CAD build for the part. Positions are in the model's coordinates, mm. A direction names the side the tool comes from. Give positions to 0.01 mm unless a question says otherwise; leave off trailing zeros. Loops run counter-clockwise (first coordinate to the right, second up) from the corner with the lowest first, then second, coordinate; pieces in that order, holes last.
Item 1: Drop flat-ended pins along their axis: P1, Ø1, axis at y = 27, z = -35, coming from the -X side; P2, Ø12, axis at x = 11, y = 132.5, coming from the -Z side; P3, Ø8, axis at x = 11, y = 55, coming from the -Z side. Give the stop position or say it passes through.
Item 2: Probe probe 1 along X at (y, z) = (36, -101.5); probe 2 along Z at (x, y) = (22, 121); probe 3 along Z at (x, y) = (11, 14.5). List the from-to ranges inside material, lowest first.
Item 3: Saw through at A-A on x = 14.25. Give the cut face in (y, z).
Item 4: Saw through at C-C on z = -15. Give the cut face in (x, y).
Item 5: Saw through at D-D on y = 35. Give the cut face in (x, z), plus the area to 3 significant figures.
Item 6: Which spindle directions (+Z, -Z, +X, -X, +Y, -Y) get a long thin tool onto all of the face, cutting with end or side? Do faces 1 (the cylindrical face through (14.93, 7.796, -116.484)), 2 (the flat face through (5, 99, -10)), 3 (the flat face through (20, 79, -51)). Say none if no direction does.
Item 7: Saw through at B-B on y = 103. Give the cut face in (x, z), plus the area to 3 significant figures.
from build123d import *

# Parameters (mm, degrees)
RESSALTO_EXTRUS_O1_DEPTH = 30
ESBO_O7_W                = 124.831233659
ESBO_O7_H                = 205.409079033
CORTE_EXTRUS_O1_DEPTH    = 26
ESBO_O9_W                = 108.1037386
ESBO_O9_H                = 206.486977543
CORTE_EXTRUS_O2_DEPTH    = 72


with BuildPart() as part:
    # Esboço1 → Ressalto-extrusão1 (new body)
    with BuildSketch(Plane(origin=(0, 0, 0), x_dir=(0, 0, -1), z_dir=(1, 0, 0))):
        with BuildLine():
            Line((0, 0), (0, 200))
            Line((0, 200), (40.020408359, 200))
            ThreePointArc((40.020408359, 200), (48.108078735, 195.725277713), (53.718695877, 188.5))
            Line((53.718695877, 188.5), (64.817635807, 160.769350553))
            Line((64.817635807, 160.769350553), (115.921293578, 17.653015861))
            ThreePointArc((115.921293578, 17.653015861), (116.438632656, 7.659898466), (110, 0))
            Line((110, 0), (0, 0))
        make_face()
    extrude(amount=RESSALTO_EXTRUS_O1_DEPTH)

    # Esboço7 → Corte-extrusão1 (cut)
    with BuildSketch(Plane(origin=(20, 0, 0), x_dir=(0, 0, -1), z_dir=(1, 0, 0))):
        with Locations((72.41561683, 101.939412441)):
            Rectangle(ESBO_O7_W, ESBO_O7_H)
    extrude(amount=CORTE_EXTRUS_O1_DEPTH, mode=Mode.SUBTRACT)

    # Esboço9 → Corte-extrusão2 (cut)
    with BuildSketch(Plane.ZY.offset(-10)):
        with Locations((-64.0518693, 99.930966914)):
            Rectangle(ESBO_O9_W, ESBO_O9_H)
    extrude(amount=CORTE_EXTRUS_O2_DEPTH, mode=Mode.SUBTRACT)


solid = part.part
Results below:
1. P1: stops at x = 10
1. P2: stops at z = -77.05
1. P3: stops at z = -104.01
2. probe 1: x = 10 to 20
2. probe 2: z = -10 to 0
2. probe 3: z = -116.92 to 0
3. outline: (0, -110) arc R13.65 ccw to (17.65, -115.92) - (160.77, -64.82) - (188.5, -53.72) arc R21.72 ccw to (200, -40.02) - (200, 0) - (0, 0) - close
4. outline: (10, 0) - (20, 0) - (20, 200) - (10, 200) - close
5. outline: (0, -10) - (10, -10) - (10, -109.73) - (20, -109.73) - (20, -10) - (30, -10) - (30, 0) - (0, 0) - close
5. area: 1,300 mm2
6. face 1: -Z, +X, -X
6. face 2: -Z, -X, +Y, -Y
6. face 3: -Z, +X, +Y, -Y
7. outline: (0, -10) - (10, -10) - (10, -85.45) - (20, -85.45) - (20, -10) - (30, -10) - (30, 0) - (0, 0) - close
7. area: 1,050 mm2
